For this review, use the dimensioned drawing (mm, ordinates from the lowest corner) and the shaded views. A direction names the side the tool comes from. Round coordinates to 2 decimals unless told otherwise and drop trailing zeros. Write each loop counter-clockwise with the first axis right and the second up, starting at its lowest first coordinate (ties: lowest second). Pieces come first, ordered by that corner, then holes. Notation, with made-up numbers: (12, -37) -> (16, -37) arc R12 ccw to (16, -30) -> close; hole circle Ø6 at (-39, 22.5). An arc over 180 degrees is marked (long way). Write each question's results on one line, items separated by ' | '. Start each with the question number.
Item 1: Clearance check with flat-ended pins moving along their axes: pin 1 (4 mm diameter, centred on x = 5, z = 6, fed in from -Y); pin 2 (1.1 mm diameter, centred on x = 11, y = 10.5, fed in from -Z); pin 3 (2.5 mm diameter, centred on x = 7, y = 10.5, fed in from -Z). State where each tip first meets the part, or that it passes through.
Item 2: Add section C-C (y = 9.25). State the section outline as (x, z) points.
Item 3: Add section A-A (x = 9.25). State the section outline as (y, z) points, plus the area to 3 significant figures.
Item 4: The part is to be moulded in two halves that separate along Z. For the marked faces 4, 5 and 6, say which applies: +Z half, -Z half, draft (parallel to the pull), parting line (faces both ways), or undercut.
Item 5: Add section D-D (z = 4.5). State the section outline as (x, y) points, plus the area to 3 significant figures.
Item 6: Add section B-B (z = 1.9). State the section outline as (x, y) points, plus the area to 3 significant figures.
Item 7: Tool access review of the marked faces 1, 2 and 3: name each direction out of +Z, -Z, +X, -X, +Y, -Y from which nothing blocks a thin tool from reaching the whole face with its end or side.
Item 8: To check wall thickness, follow line 1 along Y through (x, z) = (9.1, 1.9); line 2 along X through (y, z) = (6.75, 3.75); line 3 along Z through (x, y) = (12.75, 5.25). State the ranges of each line that lie inside material, in increasing order.
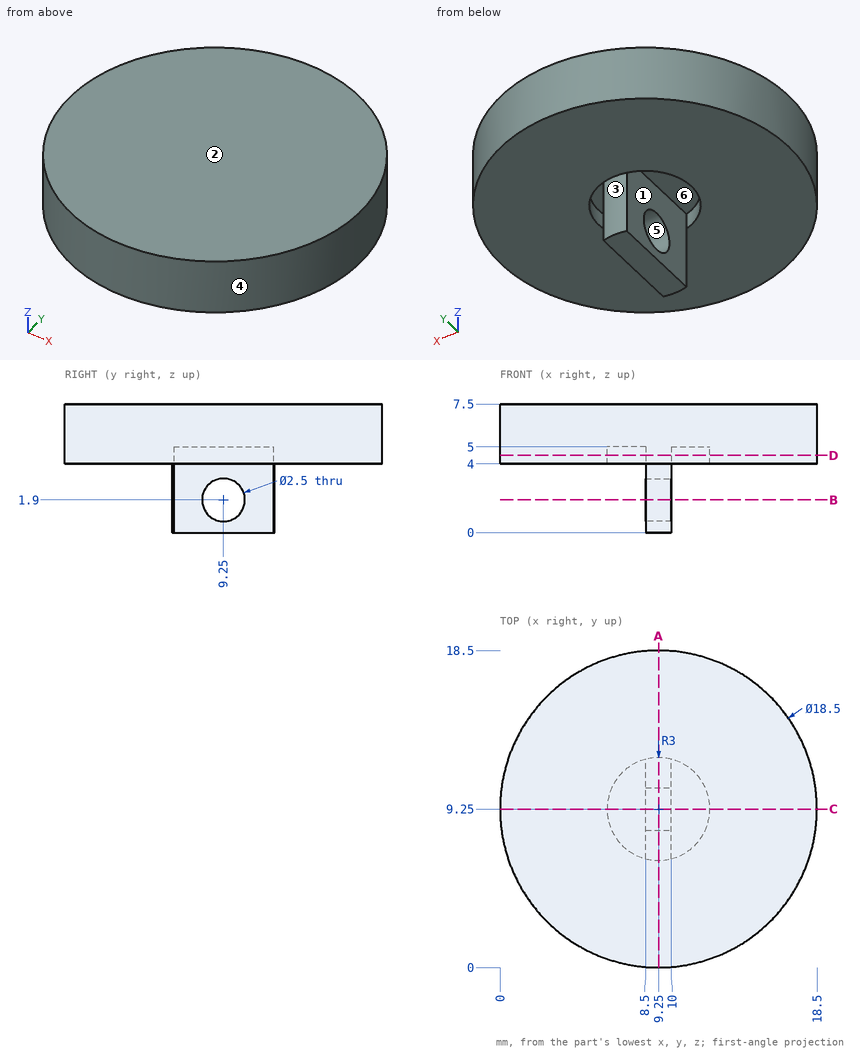
Responses:
1) pin 1: stops at y = 0.28 | pin 2: stops at z = 5 | pin 3: stops at z = 4
2) outline: (0, 4) -> (6.25, 4) -> (6.25, 5) -> (8.5, 5) -> (8.5, 3.15) -> (10, 3.15) -> (10, 5) -> (12.25, 5) -> (12.25, 4) -> (18.5, 4) -> (18.5, 7.5) -> (0, 7.5) -> close; (8.5, 0) -> (10, 0) -> (10, 0.65) -> (8.5, 0.65) -> close
3) outline: (0, 4) -> (6.25, 4) -> (6.25, 0) -> (12.25, 0) -> (12.25, 4) -> (18.5, 4) -> (18.5, 7.5) -> (0, 7.5) -> close; hole circle Ø2.5 at (9.25, 1.9) | area: 83.8 mm^2
4) face 4: draft | face 5: undercut | face 6: -Z half
5) outline: circle Ø18.5 at (9.25, 9.25); hole (8.5, 6.35) -> (8.5, 12.15) arc R3 ccw to start; hole (10, 6.35) arc R3 ccw to (10, 12.15) -> close | area: 249 mm^2
6) outline: (8.5, 6.35) arc R3 ccw to (10, 6.35) -> (10, 8) -> (8.5, 8) -> close; (8.5, 10.5) -> (10, 10.5) -> (10, 12.15) arc R3 ccw to (8.5, 12.15) -> close | area: 5.16 mm^2
7) face 1: -Z | face 2: +Z, +X, -X, +Y, -Y | face 3: -Z, +Y
8) line 1: y = 6.25 to 8, 10.5 to 12.25 | line 2: x = 8.5 to 10 | line 3: z = 4 to 7.5
